The figure shows three views and two pictorial views of one solid part (mm, origin at its lowest corner). Answer the questions. A direction names the side the tool comes from. Coordinates: 2 decimals unless noted, no trailing zeros. Loops run counter-clockwise (first coordinate to the right, second up) from the corner with the lowest first, then second, coordinate; pieces in that order, holes last. Notation, with made-up numbers: M 16.5,-11.5 L 54.5,-11.5 A25 ccw 54.5,23.5 Z; hole C -9.75,-17.75 d10. An arc over 180 degrees is marked long. Answer as a JSON object with one key per item and string values. Group by question number.
1. Straight lines are drawn through the part: L1, parallel to Z at x = 12.5, y = 2.5; L2, parallel to Z at x = 12.5, y = 10.6. For each, find the intervals that lie inside material, in ascending order.
2. Given pin 1 (1.6 mm diameter, centred on y = 12, z = 12.5, fed in from -X); pin 2 (0.6 mm diameter, centred on x = 13.5, y = 12, fed in from +Z); pin 3 (2 mm diameter, centred on y = 12, z = 8, fed in from -X), each flat-ended and moving along its own axis, determine where each tip first touches the part or whether it passes through.
3. A cutting plane is placed at D-D on y = 8. Give the vertices of the cut face in (x, z).
4. A cutting plane is placed at A-A on y = 12.75. Give the vertices of the cut face in (x, z).
5. A cutting plane is placed at C-C on z = 16. Give the vertices of the cut face in (x, y).
6. For the marked faces 1, 2 and 3, determine the directions among +Z, -Z, +X, -X, +Y, -Y from which every point of the face is accessible in a straight line to the end or side of a thin tool.
7. A cutting plane is placed at B-B on x = 12.5. Give the vertices of the cut face in (y, z).
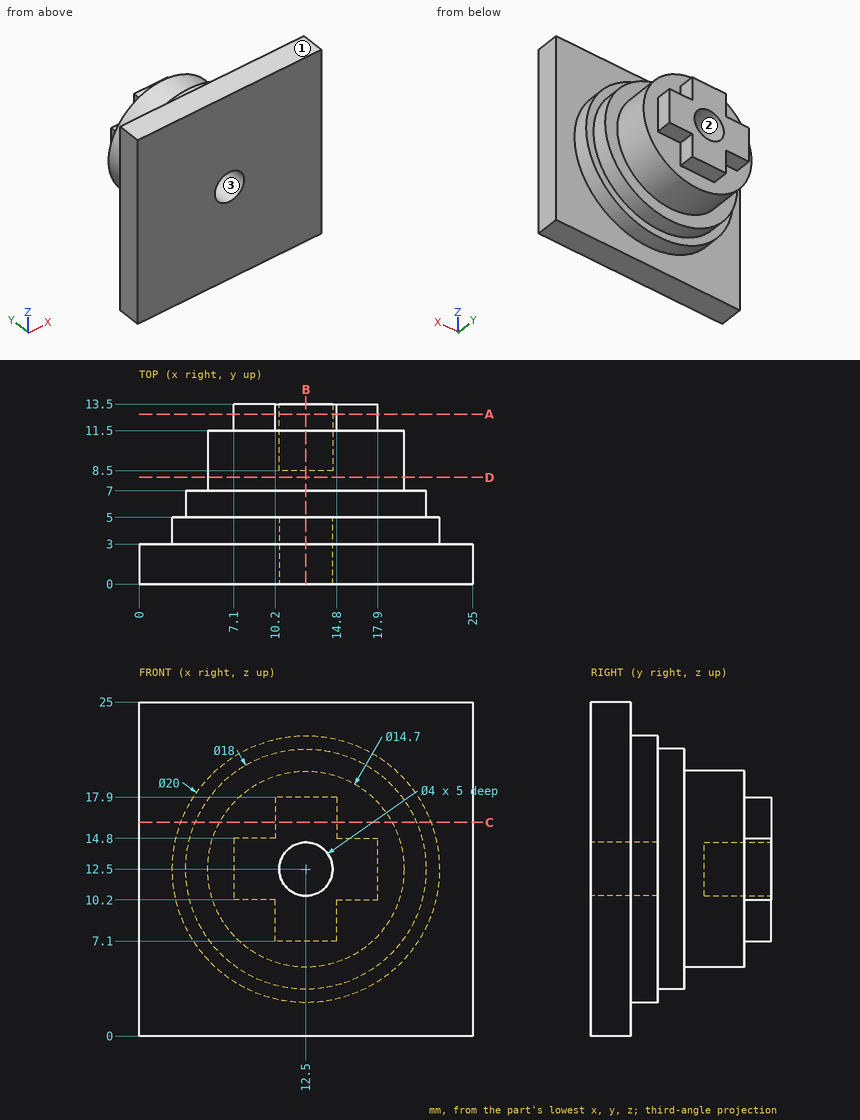
From the geometry:
{
 "1": {"L1": "z = 0 to 10.5, 14.5 to 25", "L2": "z = 5.15 to 10.5, 14.5 to 19.85"},
 "2": {"pin 1": "stops at x = 5.15", "pin 2": "stops at z = 17.9", "pin 3": "stops at x = 6.11"},
 "3": {"outline": "C 12.5,12.5 d14.7"},
 "4": {"outline": "M 7.1,10.2 L 10.2,10.2 L 10.2,7.1 L 14.8,7.1 L 14.8,10.2 L 17.9,10.2 L 17.9,14.8 L 14.8,14.8 L 14.8,17.9 L 10.2,17.9 L 10.2,14.8 L 7.1,14.8 Z; hole C 12.5,12.5 d4"},
 "5": {"outline": "M 0,0 L 25,0 L 25,3 L 21.87,3 L 21.87,5 L 20.79,5 L 20.79,7 L 18.96,7 L 18.96,11.5 L 14.8,11.5 L 14.8,13.5 L 10.2,13.5 L 10.2,11.5 L 6.04,11.5 L 6.04,7 L 4.21,7 L 4.21,5 L 3.13,5 L 3.13,3 L 0,3 Z"},
 "6": {"face 1": "+Z, +X, -X, +Y, -Y", "face 2": "+Y", "face 3": "-Y"},
 "7": {"outline": "M 0,0 L 3,0 L 3,2.5 L 5,2.5 L 5,3.5 L 7,3.5 L 7,5.15 L 11.5,5.15 L 11.5,7.1 L 13.5,7.1 L 13.5,10.5 L 8.5,10.5 L 8.5,14.5 L 13.5,14.5 L 13.5,17.9 L 11.5,17.9 L 11.5,19.85 L 7,19.85 L 7,21.5 L 5,21.5 L 5,22.5 L 3,22.5 L 3,25 L 0,25 L 0,14.5 L 5,14.5 L 5,10.5 L 0,10.5 Z"}
}
